CAD build for the part. Positions are in the model's coordinates, mm. Round coordinates to 2 decimals unless told otherwise and drop trailing zeros. Write each loop counter-clockwise with the first axis right and the second up, starting at its lowest first coordinate (ties: lowest second). Pieces come first, ordered by that corner, then holes. Notation, with made-up numbers: (-4.75, 76.25) -> (18.25, 76.25) arc R28 cw to (18.25, 102.25) -> close; hole circle Ø2 at (-38, 19.25). An arc over 180 degrees is marked (long way). Put each result on its own line as item: value. Start each with the question number.
1. Saw through at A-A on y = 25.4. List the corners of the cut face in (x, z) (3 decimals), and give its area (3 significant figures).
2. Drill centre lines: line 1 (X direction, y = 22.5, z = 1.2) (3 decimals); line 2 (Y direction, x = 44.5, z = 1.05); line 3 (Y direction, x = 15, z = 0.7). Where is each one in solid material? Low to high. Write a range as from..to.
3. Saw through at B-B on z = 0.6. List the corners of the cut face in (x, y) (1 decimal).
from build123d import *

# Parameters (mm, degrees)
SKETCH1_W           = 60.325
SKETCH1_H           = 50.8
BOSS_EXTRUDE1_DEPTH = 1.27
SKETCH3_R           = 3.2639
CUT_EXTRUDE1_DEPTH  = 2.27
CHAMFER1_SIZE       = 3.175
FILLET1_R           = 1.27


with BuildPart() as part:
    # Sketch1 → Boss-Extrude1 (new body)
    with BuildSketch(Plane.XY):
        with Locations((30.1625, 25.4)):
            Rectangle(SKETCH1_W, SKETCH1_H)
    extrude(amount=BOSS_EXTRUDE1_DEPTH)

    # Sketch3 → Cut-Extrude1 (cut, through all)
    with BuildSketch(Plane.XY.offset(1.27)):
        with Locations((42.8625, 25.4)):
            Circle(SKETCH3_R)
        with Locations((17.4625, 25.4)):
            Circle(SKETCH3_R)
    extrude(amount=-CUT_EXTRUDE1_DEPTH, mode=Mode.SUBTRACT)

    # Chamfer1
    chamfer1_edges = [part.edges().sort_by_distance(p)[0] for p in [
        (0, 0, 0.635),
        (0, 50.8, 0.635),
        (60.325, 50.8, 0.635),
        (60.325, 0, 0.635),
    ]]
    chamfer(chamfer1_edges, length=CHAMFER1_SIZE)

    # Fillet1
    fillet1_edges = [part.edges().sort_by_distance(p)[0] for p in [
        (57.15, 0, 0.635),
        (3.175, 0, 0.635),
        (0, 47.625, 0.635),
        (0, 3.175, 0.635),
        (57.15, 50.8, 0.635),
        (3.175, 50.8, 0.635),
        (60.325, 3.175, 0.635),
        (60.325, 47.625, 0.635),
    ]]
    fillet(fillet1_edges, radius=FILLET1_R)


solid = part.part
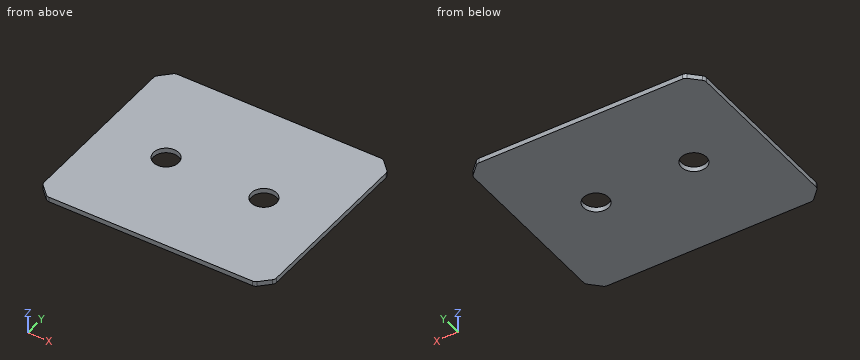
Return value:
1. outline: (0, 0) -> (14.199, 0) -> (14.199, 1.27) -> (0, 1.27) -> close; (20.726, 0) -> (39.599, 0) -> (39.599, 1.27) -> (20.726, 1.27) -> close; (46.126, 0) -> (60.325, 0) -> (60.325, 1.27) -> (46.126, 1.27) -> close
1. area: 60.0 mm^2
2. line 1: x = 0..15.965, 18.96..41.365, 44.36..60.325
2. line 2: y = 0..22.58, 28.22..50.8
2. line 3: y = 0..23.26, 27.54..50.8
3. outline: (0, 3.7) arc R1.3 ccw to (0.4, 2.8) -> (2.8, 0.4) arc R1.3 ccw to (3.7, 0) -> (56.6, 0) arc R1.3 ccw to (57.5, 0.4) -> (60, 2.8) arc R1.3 ccw to (60.3, 3.7) -> (60.3, 47.1) arc R1.3 ccw to (60, 48) -> (57.5, 50.4) arc R1.3 ccw to (56.6, 50.8) -> (3.7, 50.8) arc R1.3 ccw to (2.8, 50.4) -> (0.4, 48) arc R1.3 ccw to (0, 47.1) -> close; hole circle Ø6.5 at (17.5, 25.4); hole circle Ø6.5 at (42.9, 25.4)
